from build123d import *

# Parameters (mm, degrees)
SKETCH1_R           = 1.65
SKETCH1_R_2         = 11.5
BOSS_EXTRUDE1_DEPTH = 7
CUT_EXTRUDE3_DEPTH  = 3
BOSS_EXTRUDE4_START = -27
BOSS_EXTRUDE4_DEPTH = 27
CUT_EXTRUDE4_DEPTH  = 20
SKETCH7_R           = 2.2
CUT_EXTRUDE5_DEPTH  = 27
SKETCH8_R           = 3.5
CUT_EXTRUDE6_DEPTH  = 2
CUT_EXTRUDE7_START  = -8
SKETCH9_R           = 2.2
CUT_EXTRUDE7_DEPTH  = 8
CUT_EXTRUDE8_START  = -2
SKETCH10_R          = 3.5
CUT_EXTRUDE8_DEPTH  = 2
SKETCH11_R          = 3.5
CUT_EXTRUDE9_DEPTH  = 2
SKETCH12_R          = 1.6
CUT_EXTRUDE10_DEPTH = 7


with BuildPart() as part:
    # Sketch1 → Boss-Extrude1 (new body)
    with BuildSketch(Plane(origin=(0, 0, 0), x_dir=(1, 0, 0), z_dir=(0, 1, 0))):
        with BuildLine():
            Line((-35.480538417, 14.828911565), (-3.480538417, 14.828911565))
            ThreePointArc((-3.480538417, 14.828911565), (0.054995489, 13.364445471), (1.519461583, 9.828911565))
            Line((1.519461583, 9.828911565), (1.519461583, -22.171088435))
            ThreePointArc((1.519461583, -22.171088435), (0.054995489, -25.706622341), (-3.480538417, -27.171088435))
            Line((-3.480538417, -27.171088435), (-35.480538417, -27.171088435))
            ThreePointArc((-35.480538417, -27.171088435), (-39.016072323, -25.706622341), (-40.480538417, -22.171088435))
            Line((-40.480538417, -22.171088435), (-40.480538417, 9.828911565))
            ThreePointArc((-40.480538417, 9.828911565), (-39.016072323, 13.364445471), (-35.480538417, 14.828911565))
        make_face()
        with Locations(Location((-34.980538417, 9.328911565, 0), (0, 0, 270))):
            Circle(SKETCH1_R, mode=Mode.SUBTRACT)
        with Locations(Location((-3.980538417, 9.328911565, 0), (0, 0, 270))):
            Circle(SKETCH1_R, mode=Mode.SUBTRACT)
        with Locations(Location((-34.980538417, -21.671088435, 0), (0, 0, 270))):
            Circle(SKETCH1_R, mode=Mode.SUBTRACT)
        with Locations(Location((-3.980538417, -21.671088435, 0), (0, 0, 270))):
            Circle(SKETCH1_R, mode=Mode.SUBTRACT)
        with Locations(Location((-19.480538417, -6.171088435, 0), (0, 0, 270))):
            Circle(SKETCH1_R_2, mode=Mode.SUBTRACT)
    extrude(amount=BOSS_EXTRUDE1_DEPTH)

    # Sketch4 → Cut-Extrude3 (cut)
    with BuildSketch(Plane.XZ):
        Polygon((-22.480538417, 27.171088435), (-16.480538417, 27.171088435), (-16.480538417, 22.439037628), (-17.980538417, 21.573012224), (-19.480538417, 20.70698682), (-22.480538417, 22.439037628), align=None)
        Polygon((1.519461583, 3.171088435), (-3.212589224, 3.171088435), (-4.078614628, 4.671088435), (-4.944640032, 6.171088435), (-3.212589224, 9.171088435), (1.519461583, 9.171088435), align=None)
        Polygon((-22.480538417, -14.828911565), (-22.480538417, -10.096860757), (-20.980538417, -9.230835353), (-19.480538417, -8.364809949), (-16.480538417, -10.096860757), (-16.480538417, -14.828911565), align=None)
        Polygon((-40.480538417, 9.171088435), (-35.748487609, 9.171088435), (-34.882462206, 7.671088435), (-34.016436802, 6.171088435), (-35.748487609, 3.171088435), (-40.480538417, 3.171088435), align=None)
    extrude(amount=-CUT_EXTRUDE3_DEPTH, mode=Mode.SUBTRACT)

    # Sketch5 → Boss-Extrude4 (add)
    with BuildSketch(Plane(origin=(0, 7, 0), x_dir=(1, 0, 0), z_dir=(0, 1, 0)).offset(BOSS_EXTRUDE4_START)):
        with BuildLine():
            Line((-47.480538417, 9.828911565), (-47.480538417, -22.171088435))
            ThreePointArc((-47.480538417, -22.171088435), (-43.965819791, -30.65636981), (-35.480538417, -34.171088435))
            Line((-35.480538417, -34.171088435), (-3.480538417, -34.171088435))
            ThreePointArc((-3.480538417, -34.171088435), (5.004742957, -30.65636981), (8.519461583, -22.171088435))
            Line((8.519461583, -22.171088435), (8.519461583, 9.828911565))
            ThreePointArc((8.519461583, 9.828911565), (5.004742957, 18.314192939), (-3.480538417, 21.828911565))
            Line((-3.480538417, 21.828911565), (-35.480538417, 21.828911565))
            ThreePointArc((-35.480538417, 21.828911565), (-43.965819791, 18.314192939), (-47.480538417, 9.828911565))
        make_face()
        with BuildLine():
            ThreePointArc((-35.480538417, 14.828911565), (-39.016072323, 13.364445471), (-40.480538417, 9.828911565))
            Line((-40.480538417, 9.828911565), (-40.480538417, -22.171088435))
            ThreePointArc((-40.480538417, -22.171088435), (-39.016072323, -25.706622341), (-35.480538417, -27.171088435))
            Line((-35.480538417, -27.171088435), (-3.480538417, -27.171088435))
            ThreePointArc((-3.480538417, -27.171088435), (0.054995489, -25.706622341), (1.519461583, -22.171088435))
            Line((1.519461583, -22.171088435), (1.519461583, 9.828911565))
            ThreePointArc((1.519461583, 9.828911565), (0.054995489, 13.364445471), (-3.480538417, 14.828911565))
            Line((-3.480538417, 14.828911565), (-35.480538417, 14.828911565))
        make_face(mode=Mode.SUBTRACT)
    extrude(amount=BOSS_EXTRUDE4_DEPTH)

    # Sketch6 → Cut-Extrude4 (cut)
    with BuildSketch(Plane.XZ.offset(20)):
        with BuildLine():
            Line((2.119461583, 22.271088435), (2.119461583, -9.928911565))
            ThreePointArc((2.119461583, -9.928911565), (0.50854888, -13.817998861), (-3.380538417, -15.428911565))
            Line((-3.380538417, -15.428911565), (-35.580538417, -15.428911565))
            ThreePointArc((-35.580538417, -15.428911565), (-39.469625713, -13.817998861), (-41.080538417, -9.928911565))
            Line((-41.080538417, -9.928911565), (-41.080538417, 22.271088435))
            ThreePointArc((-41.080538417, 22.271088435), (-39.469625713, 26.160175732), (-35.580538417, 27.771088435))
            Line((-35.580538417, 27.771088435), (-3.380538417, 27.771088435))
            ThreePointArc((-3.380538417, 27.771088435), (0.50854888, 26.160175732), (2.119461583, 22.271088435))
        make_face()
    extrude(amount=-CUT_EXTRUDE4_DEPTH, mode=Mode.SUBTRACT)

    # Sketch7 → Cut-Extrude5 (cut)
    with BuildSketch(Plane.ZY.offset(-2.119461583)):
        with Locations((-1.878911565, -10)):
            Circle(SKETCH7_R)
        with Locations((14.221088435, -10)):
            Circle(SKETCH7_R)
    extrude(amount=-CUT_EXTRUDE5_DEPTH, mode=Mode.SUBTRACT)

    # Sketch8 → Cut-Extrude6 (cut)
    with BuildSketch(Plane.ZY.offset(-2.119461583)):
        with Locations((-1.878911565, -10)):
            Circle(SKETCH8_R)
        with Locations((14.221088435, -10)):
            Circle(SKETCH8_R)
    extrude(amount=-CUT_EXTRUDE6_DEPTH, mode=Mode.SUBTRACT)

    # Sketch9 → Cut-Extrude7 (cut)
    with BuildSketch(Plane(origin=(-41.080538417, 0, 0), x_dir=(0, 0, -1), z_dir=(1, 0, 0)).offset(CUT_EXTRUDE7_START)):
        with Locations(Location((-14.221088435, -10, 0), (0, 0, 180))):
            Circle(SKETCH9_R)
        with Locations(Location((1.878911565, -10, 0), (0, 0, 180))):
            Circle(SKETCH9_R)
    extrude(amount=CUT_EXTRUDE7_DEPTH, mode=Mode.SUBTRACT)

    # Sketch10 → Cut-Extrude8 (cut)
    with BuildSketch(Plane(origin=(-41.080538417, 0, 0), x_dir=(0, 0, -1), z_dir=(1, 0, 0)).offset(CUT_EXTRUDE8_START)):
        with Locations(Location((-14.221088435, -10, 0), (0, 0, 180))):
            Circle(SKETCH10_R)
        with Locations(Location((1.878911565, -10, 0), (0, 0, 180))):
            Circle(SKETCH10_R)
    extrude(amount=CUT_EXTRUDE8_DEPTH, mode=Mode.SUBTRACT)

    # Sketch11 → Cut-Extrude9 (cut)
    with BuildSketch(Plane(origin=(0, 7, 0), x_dir=(1, 0, 0), z_dir=(0, 1, 0))):
        with Locations(Location((-34.980538417, 9.328911565, 0), (0, 0, 270))):
            Circle(SKETCH11_R)
        with Locations(Location((-3.980538417, 9.328911565, 0), (0, 0, 270))):
            Circle(SKETCH11_R)
        with Locations(Location((-34.980538417, -21.671088435, 0), (0, 0, 270))):
            Circle(SKETCH11_R)
        with Locations(Location((-3.980538417, -21.671088435, 0), (0, 0, 270))):
            Circle(SKETCH11_R)
    extrude(amount=-CUT_EXTRUDE9_DEPTH, mode=Mode.SUBTRACT)

    # Sketch12 → Cut-Extrude10 (cut)
    with BuildSketch(Plane(origin=(0, 7, 0), x_dir=(1, 0, 0), z_dir=(0, 1, 0))):
        with Locations(Location((-19.480538417, 11.828911565, 0), (0, 0, 270))):
            Circle(SKETCH12_R)
        with Locations(Location((-37.480538417, -6.171088435, 0), (0, 0, 270))):
            Circle(SKETCH12_R)
        with Locations(Location((-19.480538417, -24.171088435, 0), (0, 0, 270))):
            Circle(SKETCH12_R)
        with Locations(Location((-1.480538417, -6.171088435, 0), (0, 0, 270))):
            Circle(SKETCH12_R)
    extrude(amount=-CUT_EXTRUDE10_DEPTH, mode=Mode.SUBTRACT)


solid = part.part
For this review, take the finished solid that the model builds, in its own axes (mm). A direction names the side the tool comes from. Give positions to 0.01 mm unless a question says otherwise; leave off trailing zeros. Loops run counter-clockwise (first coordinate to the right, second up) from the corner with the lowest first, then second, coordinate; pieces in that order, holes last. Notation, with made-up numbers: M -12,42.25 L 12,42.25 A15 cw 12,62.25 Z; hole C 64,37 d6. An arc over 180 degrees is marked long. Put each result on its own line as item: value. Start each with the question number.
(1) Add section D-D, the plane y = -10. Give the number of separate pieces and of enclosed holes in the cut face, then the cut area to 3 significant figures.
(2) For pin 1 (9 mm diameter, centred on y = -10, z = 14.22, fed in from -X); pin 2 (3.5 mm diameter, centred on y = -10, z = 14.22, fed in from -X); pin 3 (5 mm diameter, centred on y = -6, z = -13.5, fed in from -X); pin 4 (1.5 mm diameter, centred on x = -37.5, z = 19, fed in from -Y), all flat-tipped, find the tip position at first contact; note any pin that passes through.
(3) Add section A-A, the plane y = -2. Write out the cut boundary in (x, z), then the cut area to 3 significant figures.
(4) Add section B-B, the plane x = -29. Write out the cut boundary in (y, z), then the cut area to 3 significant figures.
(5) Wall thickness on L1, parallel to X at y = -19, z = 14.5; L2, parallel to Z at x = -27.5, y = -14.75; L3, parallel to Z at x = -4.5, y = 0.5 (3 decimals): over which ranges is each line inside the solid? List them lowest first.
(6) The part is to be moulded in two halves that separate along Z. For faces 4 (the flat face through (3, -20, 8)), 5 (the cylindrical face through (-43.87, -6.69, -18.41)), 6 (the cylindrical face through (-45.31, -11.49, -3.5)), say which applies: +Z half, -Z half, draft (parallel to the pull), parting line (faces both ways), or undercut.
(7) Add section C-C, the plane z = -6.5. Write out the cut boundary in (x, y), then the cut area to 3 significant figures.
(8) Machinability: for faces 1 (the flat face through (-20, 1, 27.171)), 2 (the cylindrical face through (-4.98, 2.46, 20.36)), 3 (the flat face through (-2, 5, -9)), which of the approach directions +Z, -Z, +X, -X, +Y, -Y give a long, thin tool a straight path to every point of the face, cutting with its end or side? Answer none if there is none.
Result:
1. separate pieces: 4
1. enclosed holes: 0
1. area: 1,040 mm^2
2. pin 1: stops at x = -47.48
2. pin 2: passes through
2. pin 3: stops at x = -47.42
2. pin 4: stops at y = 0
3. outline: M -47.48,-9.83 A12 ccw -35.48,-21.83 L -3.48,-21.83 A12 ccw 8.52,-9.83 L 8.52,22.17 A12 ccw -3.48,34.17 L -35.48,34.17 A12 ccw -47.48,22.17 Z; hole M -41.08,-9.93 A5.5 ccw -35.58,-15.43 L -3.38,-15.43 A5.5 ccw 2.12,-9.93 L 2.12,22.27 A5.5 ccw -3.38,27.77 L -35.58,27.77 A5.5 ccw -41.08,22.27 Z
3. area: 1,170 mm^2
4. outline: M -20,-21.83 L 7,-21.83 L 7,-0.28 L 0,-0.28 L 0,-15.43 L -20,-15.43 Z; M -20,27.77 L 0,27.77 L 0,12.62 L 7,12.62 L 7,34.17 L -20,34.17 Z
4. area: 558 mm^2
5. L1: x = -47.48 to -41.08, 2.12 to 8.52
5. L2: z = -21.83 to -15.43, 27.77 to 34.17
5. L3: z = -21.829 to -10.895, -7.763 to 5.401, 6.941 to 20.105, 23.237 to 34.171
6. face 4: draft
6. face 5: -Z half
6. face 6: undercut
7. outline: M -47.48,-20 L -41.08,-20 L -41.08,0 L 2.12,0 L 2.12,-20 L 8.52,-20 L 8.52,7 L -1.92,7 L -1.92,5 L -6.04,5 L -6.04,7 L -32.92,7 L -32.92,5 L -37.04,5 L -37.04,7 L -47.48,7 Z
7. area: 632 mm^2
8. face 1: -Y
8. face 2: +Y, -Y
8. face 3: +Y
